Build history of the part. All positions in model axes, mm. A direction names the side the tool comes from. Coordinates: 2 decimals unless noted, no trailing zeros. Order: outer loops, then holes, each group sorted by start corner. A loop starts at its lowest first (then second) coordinate and runs counter-clockwise, first axis right, second up. Notation, with made-up numbers: (50.25, 58) - (89.25, 58) arc R19 cw to (89.25, 64) - close; hole circle Ø8 at (62.5, 24). An arc over 180 degrees is marked (long way). Return JSON: item names as keys, results as strings.
from build123d import *

# Parameters (mm, degrees)
BOSS_EXTRUDE1_DEPTH            = 4
CUT_EXTRUDE1_DEPTH             = 5
CUT_EXTRUDE1_DEPTH_BACK        = 1
SKETCH1_6_R                    = 10
CUT_EXTRUDE2_DEPTH             = 1.93
CUT_EXTRUDE2_DEPTH_BACK        = 1
M2_5_CLEARANCE_HOLE1_D         = 2.9
CHAMFER1_SIZE                  = 0.25
BOSS_EXTRUDE5_DEPTH            = 4
SKETCH4_5_R                    = 4
BOSS_EXTRUDE6_DEPTH            = 10
TAP_DRILL_FOR_M2_5X0_45_TAP2_D = 2.05
BOSS_EXTRUDE7_DEPTH            = 1.5
MIRROR4_COPY_1_DEPTH           = 1.5
CHAMFER3_SIZE                  = 0.5


with BuildPart() as part:
    # Sketch1 → Boss-Extrude1 (new body)
    with BuildSketch(Plane.XY):
        with BuildLine():
            ThreePointArc((16.285714286, -3.282607227), (18, 0), (16.285714286, 3.282607227))
            Line((16.285714286, 3.282607227), (6.857142857, 9.84782168))
            ThreePointArc((6.857142857, 9.84782168), (0, 12), (-6.857142857, 9.84782168))
            Line((-6.857142857, 9.84782168), (-16.285714286, 3.282607227))
            ThreePointArc((-16.285714286, 3.282607227), (-18, 0), (-16.285714286, -3.282607227))
            Line((-16.285714286, -3.282607227), (-6.857142857, -9.84782168))
            ThreePointArc((-6.857142857, -9.84782168), (0, -12), (6.857142857, -9.84782168))
            Line((6.857142857, -9.84782168), (16.285714286, -3.282607227))
        make_face()
    extrude(amount=BOSS_EXTRUDE1_DEPTH)

    # Sketch1_4 → Cut-Extrude1 (cut, two sides)
    with BuildSketch(Plane.XY) as cut_extrude1_sk:
        with BuildLine():
            ThreePointArc((-8.25, 0), (0, -8.25), (8.25, 0))
            Line((8.25, 0), (-8.25, 0))
        make_face()
        with BuildLine():
            Line((-8.25, 0), (8.25, 0))
            ThreePointArc((8.25, 0), (0, 8.25), (-8.25, 0))
        make_face()
    extrude(amount=CUT_EXTRUDE1_DEPTH, mode=Mode.SUBTRACT)
    extrude(cut_extrude1_sk.sketch, amount=-CUT_EXTRUDE1_DEPTH_BACK, mode=Mode.SUBTRACT)

    # Sketch1_6 → Cut-Extrude2 (cut, two sides)
    with BuildSketch(Plane.XY) as cut_extrude2_sk:
        Circle(SKETCH1_6_R)
    extrude(amount=CUT_EXTRUDE2_DEPTH, mode=Mode.SUBTRACT)
    extrude(cut_extrude2_sk.sketch, amount=-CUT_EXTRUDE2_DEPTH_BACK, mode=Mode.SUBTRACT)

    # M2.5 Clearance Hole1 (through all)
    with Locations(Plane.XY.offset(4)):
        with Locations((-14, 0), (14, 0)):
            Hole(M2_5_CLEARANCE_HOLE1_D / 2)

    # Chamfer1
    chamfer1_edges = [part.edges().sort_by_distance(p)[0] for p in [
        (-8.25, 0, 4),
        (-10, 0, 0),
        (-10, 0, 1.93),
        (-8.25, 0, 1.93),
    ]]
    chamfer(chamfer1_edges, length=CHAMFER1_SIZE)

    # Sketch4_4 → Boss-Extrude5 (add)
    with BuildSketch(Plane.XY):
        with BuildLine():
            Line((11.172261915, 4.379562044), (3.724087305, 23.379854015))
            ThreePointArc((3.724087305, 23.379854015), (0, 25.92), (-3.724087305, 23.379854015))
            Line((-3.724087305, 23.379854015), (-11.172261915, 4.379562044))
            ThreePointArc((-11.172261915, 4.379562044), (0, 12), (11.172261915, 4.379562044))
        make_face()
        with BuildLine():
            ThreePointArc((11.172261915, -4.379562044), (0, -12), (-11.172261915, -4.379562044))
            Line((-11.172261915, -4.379562044), (-3.724087305, -23.379854015))
            ThreePointArc((-3.724087305, -23.379854015), (0, -25.92), (3.724087305, -23.379854015))
            Line((3.724087305, -23.379854015), (11.172261915, -4.379562044))
        make_face()
    extrude(amount=BOSS_EXTRUDE5_DEPTH)

    # Sketch4_5 → Boss-Extrude6 (add)
    with BuildSketch(Plane.XY):
        with Locations((0, 21.92)):
            Circle(SKETCH4_5_R)
        with Locations((0, -21.92)):
            Circle(SKETCH4_5_R)
    extrude(amount=BOSS_EXTRUDE6_DEPTH)

    # Tap Drill for M2.5x0.45 Tap2 (through all)
    with Locations(Plane.XY.offset(10)):
        with Locations((0, 21.92), (0, -21.92)):
            Hole(TAP_DRILL_FOR_M2_5X0_45_TAP2_D / 2)

    # Sketch10 → Boss-Extrude7 (add)
    with BuildSketch(Plane(origin=(-11.172261915, -4.379562044, 0), x_dir=(0, 0, 1), z_dir=(-0.931021826, -0.364963504, 0))):
        Polygon((10, -20.407998432), (4, -12.407998432), (4, -20.407998432), align=None)
    boss_extrude7 = extrude(amount=-BOSS_EXTRUDE7_DEPTH)

    # Mirror3: Boss-Extrude7 across plane
    add(boss_extrude7.mirror(Plane(origin=(0, 0, 0), x_dir=(0, 0, 1), z_dir=(1, 0, 0))))

    # Mirror4: Boss-Extrude7 across plane
    add(boss_extrude7.mirror(Plane.ZX))

    # Mirror4 copy 1 sketch → Mirror4 copy 1 (add)
    with BuildSketch(Plane(origin=(11.172261915, 4.379562044, 0), x_dir=(0, 0, 1), z_dir=(0.931021826, 0.364963504, 0))):
        Polygon((10, -20.407998432), (4, -12.407998432), (4, -20.407998432), align=None)
    extrude(amount=-MIRROR4_COPY_1_DEPTH)

    # Chamfer3
    chamfer3_edges = [part.edges().sort_by_distance(p)[0] for p in [
        (1.025, -21.92, 10),
        (1.025, 21.92, 10),
    ]]
    chamfer(chamfer3_edges, length=CHAMFER3_SIZE)


solid = part.part
1. Mould opens along Y. For faces 1 (the flat face through (-4.799, -18.61, 6.375)), 2 (the flat face through (0, 20, 10)), 3 (the flat face through (-13.1, -5.5, 2)) say: pulls with the +Y half, pulls with the -Y half, needs draft (parallel to the pull), parting line crosses it, or undercut.
Check values:
{"face 1": "undercut", "face 2": "needs draft", "face 3": "pulls with the -Y half"}
2. Cut at A-A on y = 0. Give the cut face in (x, z).
Check values:
{"outline": "(-18, 0) - (-15.45, 0) - (-15.45, 4) - (-18, 4) - close; (-12.55, 0) - (-10.25, 0) - (-10, 0.25) - (-10, 1.68) - (-9.75, 1.93) - (-8.5, 1.93) - (-8.25, 2.18) - (-8.25, 3.75) - (-8.5, 4) - (-12.55, 4) - close; (8.25, 2.18) - (8.5, 1.93) - (9.75, 1.93) - (10, 1.68) - (10, 0.25) - (10.25, 0) - (12.55, 0) - (12.55, 4) - (8.5, 4) - (8.25, 3.75) - close; (15.45, 0) - (18, 0) - (18, 4) - (15.45, 4) - close"}
3. Cut at D-D on y = -21.92. Give the cut face in (x, z) (3 decimals), plus the area to 3 significant figures.
Check values:
{"outline": "(-4.296, 0) - (-1.025, 0) - (-1.025, 9.5) - (-1.525, 10) - (-4, 10) - (-4, 8.905) - (-4.296, 8.824) - close; (1.025, 0) - (4.296, 0) - (4.296, 8.824) - (4, 8.905) - (4, 10) - (1.525, 10) - (1.025, 9.5) - close", "area": "64.5 mm²"}
4. Cut at B-B on z = 5.5. Give the cut face in (x, y) (3 decimals).
Check values:
{"outline": "(-5.914, -17.794) - (-3.724, -23.38) arc R4 ccw to (3.724, -23.38) - (5.914, -17.794) - (4.517, -17.246) - (3.467, -19.925) arc R4 ccw to (-3.467, -19.925) - (-4.517, -17.246) - close; (-5.914, 17.794) - (-4.517, 17.246) - (-3.467, 19.925) arc R4 ccw to (3.467, 19.925) - (4.517, 17.246) - (5.914, 17.794) - (3.724, 23.38) arc R4 ccw to (-3.724, 23.38) - close; hole circle Ø2.05 at (0, -21.92); hole circle Ø2.05 at (0, 21.92)"}
5. Cut at C-C on x = 14. Give the cut face in (y, z).
Check values:
{"outline": "(-4.87, 0) - (-1.45, 0) - (-1.45, 4) - (-4.87, 4) - close; (1.45, 0) - (4.87, 0) - (4.87, 4) - (1.45, 4) - close"}
6. Drop flat-ended pins along their axis: pin 1 (11 mm diameter, centred on x = -6.5, y = -4.5, fed in from +Z); pin 2 (2.5 mm diameter, centred on x = 0, y = 21.92, fed in from -Z). Give the stop position or say it passes through.
Check values:
{"pin 1": "z = 4", "pin 2": "z = 0"}
7. Probe L1, parallel to Y at x = -14, z = 2.15; L2, parallel to Y at x = 2, z = 5; L3, parallel to Z at x = -3, y = 9. List the from-to ranges inside material, lowest first.
Check values:
{"L1": "-4.87 to -1.45, 1.45 to 4.87", "L2": "-25.38 to -18.46, 18.46 to 25.38", "L3": "1.93 to 4"}
8. Tool access for faces 4 (the flat face through (1, 9, 1.93)), 5 (the flat face through (0, -9, 4)), 6 (the flat face through (-4.799, 18.61, 6.375)): list every direction of +Z, -Z, +X, -X, +Y, -Y with a clear straight run to the whole face (end or side of a thin tool).
Check values:
{"face 4": "-Z", "face 5": "+Z", "face 6": "+Z, -X"}
